Geometry: final body of the model. Coordinates: model frame, mm. Face numbers are marked on the shaded views. A direction names the side the tool comes from. Give positions to 0.01 mm unless a question says otherwise; leave off trailing zeros. Order: outer loops, then holes, each group sorted by start corner. A loop starts at its lowest first (then second) coordinate and runs counter-clockwise, first axis right, second up. Notation, with made-up numbers: (24.5, -24) -> (32.5, -24) arc R20 ccw to (32.5, -12) -> close; hole circle Ø5 at (47.5, 89). An arc over 180 degrees is marked (long way). One line per question, with ' | ' between items.
from build123d import *

# Parameters (mm, degrees)
SKETCH1_W           = 66
SKETCH1_H           = 5
BASE_FLANGE1_DEPTH  = 2
SKETCH2_R           = 2.5
BOSS_EXTRUDE1_DEPTH = 3
SKETCH3_W           = 2
SKETCH3_H           = 5
BOSS_EXTRUDE2_DEPTH = 11
SKETCH4_W           = 6
SKETCH4_H           = 5
BOSS_EXTRUDE3_DEPTH = 2
SKETCH5_R           = 1.5
CUT_EXTRUDE1_DEPTH  = 40.537956447
SKETCH6_R           = 1.25
CUT_EXTRUDE2_DEPTH  = 41.598645298
SKETCH7_W           = 2
SKETCH7_H           = 5
BOSS_EXTRUDE4_DEPTH = 25
BOSS_EXTRUDE5_DEPTH = 5
BOSS_EXTRUDE6_DEPTH = 8
SKETCH13_W          = 65
SKETCH13_H          = 6
BOSS_EXTRUDE8_DEPTH = 2
SKETCH12_W          = 6
SKETCH12_H          = 49
BOSS_EXTRUDE7_DEPTH = 2
SKETCH14_R          = 2.5
BOSS_EXTRUDE9_DEPTH = 2
CUT_EXTRUDE3_REACH  = 53.732
SKETCH15_R          = 1.25


# Sheet-metal steps are written as plain solids
with BuildPart() as part:
    # Sketch1 → Base-Flange1 (new body)
    with BuildSketch(Plane(origin=(0, 0, 0), x_dir=(1, 0, 0), z_dir=(0, 1, 0))):
        Rectangle(SKETCH1_W, SKETCH1_H)
    extrude(amount=-BASE_FLANGE1_DEPTH)

    # Sketch2 → Boss-Extrude1 (add)
    with BuildSketch(Plane(origin=(0, 0, 0), x_dir=(-1, 0, 0), z_dir=(0, -1, 0))):
        with Locations(Location((19.7, 0, 0), (0, 0, 90))):
            Circle(SKETCH2_R)
        with Locations(Location((-29.3, 0, 0), (0, 0, 90))):
            Circle(SKETCH2_R)
    extrude(amount=-BOSS_EXTRUDE1_DEPTH)

    # Sketch3 → Boss-Extrude2 (add)
    with BuildSketch(Plane(origin=(0, -2, 0), x_dir=(-1, 0, 0), z_dir=(0, -1, 0))):
        with Locations((-34, 0)):
            Rectangle(SKETCH3_W, SKETCH3_H)
    boss_extrude2 = extrude(amount=-BOSS_EXTRUDE2_DEPTH)

    # Sketch4 → Boss-Extrude3 (add)
    with BuildSketch(Plane(origin=(0, 9, 0), x_dir=(1, 0, 0), z_dir=(0, 1, 0))):
        with Locations((36, 0)):
            Rectangle(SKETCH4_W, SKETCH4_H)
    boss_extrude3 = extrude(amount=-BOSS_EXTRUDE3_DEPTH)

    # Mirror1: Boss-Extrude2, Boss-Extrude3 across plane
    add(boss_extrude2.mirror(Plane(origin=(0, 0, 0), x_dir=(0, 0, 1), z_dir=(1, 0, 0))))
    add(boss_extrude3.mirror(Plane(origin=(0, 0, 0), x_dir=(0, 0, 1), z_dir=(1, 0, 0))))

    # Sketch5 → Cut-Extrude1 (cut, through all)
    with BuildSketch(Plane(origin=(0, 3, 0), x_dir=(1, 0, 0), z_dir=(0, 1, 0))):
        with Locations(Location((-19.7, 0, 0), (0, 0, 270))):
            Circle(SKETCH5_R)
        with Locations(Location((29.3, 0, 0), (0, 0, 270))):
            Circle(SKETCH5_R)
    extrude(amount=-CUT_EXTRUDE1_DEPTH, mode=Mode.SUBTRACT)

    # Sketch6 → Cut-Extrude2 (cut, through all)
    with BuildSketch(Plane(origin=(0, 9, 0), x_dir=(1, 0, 0), z_dir=(0, 1, 0))):
        with Locations(Location((-37, 0, 0), (0, 0, 270))):
            Circle(SKETCH6_R)
        with Locations(Location((37, 0, 0), (0, 0, 270))):
            Circle(SKETCH6_R)
    extrude(amount=-CUT_EXTRUDE2_DEPTH, mode=Mode.SUBTRACT)

    # Sketch7 → Boss-Extrude4 (add)
    with BuildSketch(Plane(origin=(0, -2, 0), x_dir=(-1, 0, 0), z_dir=(0, -1, 0))):
        with Locations((29, 0)):
            Rectangle(SKETCH7_W, SKETCH7_H)
    boss_extrude4 = extrude(amount=BOSS_EXTRUDE4_DEPTH)

    # Sketch8 → Boss-Extrude5 (add)
    with BuildSketch(Plane.XY.offset(2.5)):
        Polygon((-28, -3), (-26, -5), (-28, -5), align=None)
        Polygon((-28, -7), (-26, -7), (-28, -9), align=None)
        Polygon((-28, -21), (-28, -23), (-26, -23), align=None)
        Polygon((-28, -25), (-28, -27), (-26, -25), align=None)
    boss_extrude5 = extrude(amount=-BOSS_EXTRUDE5_DEPTH)

    # Mirror2: Boss-Extrude4, Boss-Extrude5 across plane
    add(boss_extrude4.mirror(Plane(origin=(2.5, 0, 0), x_dir=(0, 0, 1), z_dir=(1, 0, 0))))
    add(boss_extrude5.mirror(Plane(origin=(2.5, 0, 0), x_dir=(0, 0, 1), z_dir=(1, 0, 0))))

    # Sketch11 → Boss-Extrude6 (add)
    with BuildSketch(Plane.XY.offset(-2.5)):
        Polygon((-30, -27), (-30, 0), (35, 0), (35, -27), (33, -27), (33, -2), (-28, -2), (-28, -27), align=None)
    extrude(amount=-BOSS_EXTRUDE6_DEPTH)

    # Sketch13 → Boss-Extrude8 (add)
    with BuildSketch(Plane(origin=(0, 0, -10.5), x_dir=(-1, 0, 0), z_dir=(0, 0, -1))):
        with Locations((-2.5, -24)):
            Rectangle(SKETCH13_W, SKETCH13_H)
    extrude(amount=-BOSS_EXTRUDE8_DEPTH)

    # Sketch12 → Boss-Extrude7 (add)
    with BuildSketch(Plane(origin=(0, 0, -10.5), x_dir=(-1, 0, 0), z_dir=(0, 0, -1))):
        with Locations((-21.5, -6)):
            Rectangle(SKETCH12_W, SKETCH12_H)
        with Locations((21.5, -6)):
            Rectangle(SKETCH12_W, SKETCH12_H)
    extrude(amount=-BOSS_EXTRUDE7_DEPTH)

    # Sketch14 → Boss-Extrude9 (add)
    with BuildSketch(Plane(origin=(0, 0, -10.5), x_dir=(-1, 0, 0), z_dir=(0, 0, -1))):
        with Locations(Location((-22, 16, 0), (0, 0, 180))):
            Circle(SKETCH14_R)
        with Locations(Location((22, 16, 0), (0, 0, 180))):
            Circle(SKETCH14_R)
        with Locations(Location((-22, -28, 0), (0, 0, 180))):
            Circle(SKETCH14_R)
        with Locations(Location((22, -28, 0), (0, 0, 180))):
            Circle(SKETCH14_R)
    extrude(amount=BOSS_EXTRUDE9_DEPTH)

    # Sketch15 → Cut-Extrude3 (cut, up to next)
    with BuildSketch(Plane(origin=(0, 0, -12.5), x_dir=(-1, 0, 0), z_dir=(0, 0, -1)), mode=Mode.PRIVATE) as cut_extrude3_sk1:
        with Locations((-22, 16)):
            Circle(SKETCH15_R)
    cut_extrude3_tool1 = extrude(cut_extrude3_sk1.sketch, amount=-CUT_EXTRUDE3_REACH, mode=Mode.PRIVATE) & part.part
    # Sketch15 → Cut-Extrude3 (cut, up to next)
    with BuildSketch(Plane(origin=(0, 0, -12.5), x_dir=(-1, 0, 0), z_dir=(0, 0, -1)), mode=Mode.PRIVATE) as cut_extrude3_sk2:
        with Locations(Location((22, 16, 0), (0, 0, 180))):
            Circle(SKETCH15_R)
    cut_extrude3_tool2 = extrude(cut_extrude3_sk2.sketch, amount=-CUT_EXTRUDE3_REACH, mode=Mode.PRIVATE) & part.part
    # Sketch15 → Cut-Extrude3 (cut, up to next)
    with BuildSketch(Plane(origin=(0, 0, -12.5), x_dir=(-1, 0, 0), z_dir=(0, 0, -1)), mode=Mode.PRIVATE) as cut_extrude3_sk3:
        with Locations((22, -28)):
            Circle(SKETCH15_R)
    cut_extrude3_tool3 = extrude(cut_extrude3_sk3.sketch, amount=-CUT_EXTRUDE3_REACH, mode=Mode.PRIVATE) & part.part
    # Sketch15 → Cut-Extrude3 (cut, up to next)
    with BuildSketch(Plane(origin=(0, 0, -12.5), x_dir=(-1, 0, 0), z_dir=(0, 0, -1)), mode=Mode.PRIVATE) as cut_extrude3_sk4:
        with Locations((-22, -28)):
            Circle(SKETCH15_R)
    cut_extrude3_tool4 = extrude(cut_extrude3_sk4.sketch, amount=-CUT_EXTRUDE3_REACH, mode=Mode.PRIVATE) & part.part
    add(cut_extrude3_tool1.solids().sort_by_distance((22, 16, -12.5))[0], mode=Mode.SUBTRACT)
    add(cut_extrude3_tool2.solids().sort_by_distance((-22, 16, -12.5))[0], mode=Mode.SUBTRACT)
    add(cut_extrude3_tool3.solids().sort_by_distance((-22, -28, -12.5))[0], mode=Mode.SUBTRACT)
    add(cut_extrude3_tool4.solids().sort_by_distance((22, -28, -12.5))[0], mode=Mode.SUBTRACT)


solid = part.part
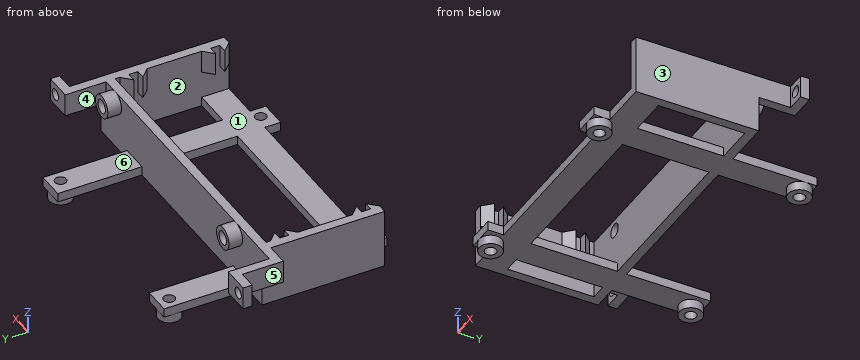
1) Material intervals for probe 1 along X at (y, z) = (0.9, 0); probe 2 along Y at (x, z) = (-22, -9.4); probe 3 along X at (y, z) = (8, 0), sorted ascending. Write a range as from..to.
Check result:
probe 1: x = -35..-33, -22.2..-21.2, -18.2..-17.2, 26.8..27.8, 30.8..31.8, 33..35 | probe 2: y = -30.5..-29.25, -26.75..14.75, 17.25..18.5 | probe 3: x = -39..-38.25, -35.75..-33, 33..35.75, 38.25..39
2) Section A-A on z = -11.25. Return loops of the section in (x, y).
Check result:
outline: circle Ø5 at (-22, -28); circle Ø5 at (-22, 16); circle Ø5 at (22, -28); circle Ø5 at (22, 16); hole circle Ø2.5 at (-22, -28); hole circle Ø2.5 at (-22, 16); hole circle Ø2.5 at (22, -28); hole circle Ø2.5 at (22, 16)
3) Set-up query: the marked faces 3, 4, 5 and 6. Return all of +Z, -Z, +X, -X, +Y, -Y with unobstructed straight access to the full face (end or side cutting, diameter ignored); none if empty.
Check result:
face 3: +Z, -Z, +X, -Y | face 4: +Z, -Z, +Y | face 5: +Z, -Z, -X, -Y | face 6: +Z, +X, -X, +Y
4) Section C-C on y = 4. Return loops of the section in (x, z).
Check result:
outline: (-35, -2.5) -> (-33, -2.5) -> (-33, 2.5) -> (-35, 2.5) -> close; (-24.5, -10.5) -> (-18.5, -10.5) -> (-18.5, -8.5) -> (-24.5, -8.5) -> close; (18.5, -10.5) -> (24.5, -10.5) -> (24.5, -8.5) -> (18.5, -8.5) -> close; (33, -2.5) -> (35, -2.5) -> (35, 2.5) -> (33, 2.5) -> close
5) Section D-D on x = -37. Return loops of the section in (y, z).
Check result:
outline: (7, -2.5) -> (9, -2.5) -> (9, -1.25) -> (7, -1.25) -> close; (7, 1.25) -> (9, 1.25) -> (9, 2.5) -> (7, 2.5) -> close
6) Section B-B on x = 14. Return loops of the section in (y, z).
Check result:
outline: (-27, -10.5) -> (-21, -10.5) -> (-21, -8.5) -> (-27, -8.5) -> close; (-2, -10.5) -> (0, -10.5) -> (0, 2.5) -> (-2, 2.5) -> close
7) Contact query for flat-ended pins moving along their axis: pin 1 Ø6 at (x, y) = (-9, -17) entering from -Z; pin 2 Ø1.5 at (y, z) = (4, 1) entering from -X; pin 3 Ø2.5 at (y, z) = (4, 0) entering from +X; pin 4 Ø0.6 at (x, y) = (32, -8) entering from -Z. Output: stop coordinate, or through.
Check result:
pin 1: passes through | pin 2: stops at x = -35 | pin 3: stops at x = 35 | pin 4: stops at z = -2.5
8) Pull-direction query (Y, two-part tool) for the marked faces 1 and 2; classes: +Y half, -Y half, draft (parallel to the pull), parting line (faces both ways), or undercut.
Check result:
face 1: draft | face 2: undercut
